Part model, mm, in its own coordinate system. Face numbers are marked on the shaded views. A direction names the side the tool comes from. Give positions to 0.01 mm unless a question says otherwise; leave off trailing zeros. Write each loop counter-clockwise with the first axis right and the second up, starting at its lowest first coordinate (ties: lowest second). Pieces come first, ordered by that corner, then holes. Notation, with made-up numbers: M 77,3 L 131,3 A19 ccw 131,37 Z; hole C -16.5,-38 d10. An arc over 180 degrees is marked long. Write item = value, one per line. Start each with the question number.
from build123d import *

# Parameters (mm, degrees)
EXTRUDE_1_DEPTH     = 20
SKETCH_2_R          = 1.5
EXTRUDE_2_DEPTH     = 4
FILLET_5_R          = 1
CUT_EXTRUDE_1_REACH = 53.828


with BuildPart() as part:
    # 草图1 → 凸台-拉伸1 (new body)
    with BuildSketch(Plane.XY):
        Polygon((20.6, 14), (24.6, 3), (24.6, -2), (20.6, -2), (20.6, 0), (14.6, 0), (14.6, 3), (17.6, 3), (17.6, 6), (14.6, 6), (14.6, 10), (6, 10), (6, 6), (3, 6), (3, 3), (6, 3), (6, 0), (0, 0), (0, 14), align=None)
    extrude(amount=EXTRUDE_1_DEPTH)

    # 草图2 → 凸台-拉伸2 (add)
    with BuildSketch(Plane(origin=(24.6, 0, 0), x_dir=(0, 0, -1), z_dir=(1, 0, 0))):
        with BuildLine():
            Line((-15, -2), (-5, -2))
            Line((-5, -2), (-5, -22))
            ThreePointArc((-5, -22), (-10, -27), (-15, -22))
            Line((-15, -22), (-15, -2))
        make_face()
        with Locations((-10, -22)):
            Circle(SKETCH_2_R, mode=Mode.SUBTRACT)
    extrude(amount=-EXTRUDE_2_DEPTH)

    # 圆角5
    fillet_5_edges = [part.edges().sort_by_distance(p)[0] for p in [
        (16.1, 3, 0),
        (17.6, 4.5, 0),
        (16.1, 6, 0),
        (4.5, 6, 0),
        (3, 4.5, 0),
        (4.5, 3, 0),
        (4.5, 3, 20),
        (3, 4.5, 20),
        (20.6, 14, 10),
        (24.6, 3, 10),
        (4.5, 6, 20),
        (16.1, 6, 20),
        (17.6, 4.5, 20),
        (16.1, 3, 20),
    ]]
    fillet(fillet_5_edges, radius=FILLET_5_R)

    # 草图3 → 切除-拉伸1 (cut, up to next)
    with BuildSketch(Plane(origin=(0, 14, 0), x_dir=(1, 0, 0), z_dir=(0, 1, 0)), mode=Mode.PRIVATE) as cut_extrude_1_sk1:
        with BuildLine():
            Line((8.449786368, -3), (8.449786368, -17))
            ThreePointArc((8.449786368, -17), (9.949786368, -18.5), (11.449786368, -17))
            Line((11.449786368, -17), (11.449786368, -3))
            ThreePointArc((11.449786368, -3), (9.949786368, -1.5), (8.449786368, -3))
        make_face()
    cut_extrude_1_tool1 = extrude(cut_extrude_1_sk1.sketch, amount=-CUT_EXTRUDE_1_REACH, mode=Mode.PRIVATE) & part.part
    add(cut_extrude_1_tool1.solids().sort_by_distance((9.949786, 14, 10))[0], mode=Mode.SUBTRACT)


solid = part.part
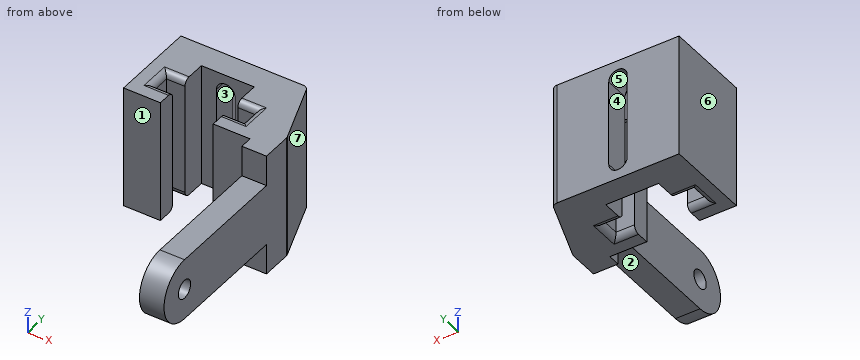
Q1. Tool access for the marked faces 1, 2 and 3: list every direction of +Z, -Z, +X, -X, +Y, -Y with a clear straight run to the whole face (end or side of a thin tool).
Q2. Probe line 1 along Y through (x, z) = (16.25, 17); line 2 along X through (y, z) = (2, 4); line 3 along Y through (x, z) = (7.5, 17). List the from-to ranges inside material, lowest first.
Q3. Drop flat-ended pins along their axis: P1, Ø1.2, axis at x = 22, z = 17.5, coming from the -Y side; P2, Ø1.8, axis at x = 3.5, z = 8.5, coming from the -Y side; P3, Ø2, axis at y = 12.5, z = 12, coming from the -X side; P4, Ø8, axis at x = 7.5, y = -6, coming from the -Z side. Give the stop position or say it passes through.
Q4. Slice it at D-D (z = 13.5). Give the cut face in (x, y), and give its area (3 significant figures).
Q5. Slice it at B-B (z = 10). Give the number of separate pieces and of enclosed holes in the cut face, and give its area (3 significant figures).
Q6. Slice it at C-C (y = 1). Give the cut face in (x, z), and give its area (3 significant figures).
Q7. Slice it at A-A (x = 15.5). Give the cut face in (y, z), and give its area (3 significant figures).
Q8. Two-plate mould, pull along X, no slides. Class the marked faces 4, 5, 6 and 7: +X half, -X half, draft (parallel to the pull), parting line (faces both ways), or undercut.
Working result:
q1.face_1 = +Z, -Z, -X, -Y
q1.face_2 = -Z, +X, -X, -Y
q1.face_3 = +Y, -Y
q2.line_1 = 0 to 3, 6 to 14
q2.line_2 = 0 to 6, 14.6 to 24.6
q2.line_3 = 10 to 14
q3.P1 = -2
q3.P2 = 0
q3.P3 = 0
q3.P4 = through
q4.outline = M 0,0 L 6,0 L 6,3 L 3,3 L 3,6 L 6,6 L 6,10 L 8.45,10 L 8.45,14 L 0,14 Z; M 11.45,10 L 14.6,10 L 14.6,6 L 17.6,6 L 17.6,3 L 14.6,3 L 14.6,0 L 20.6,0 L 20.6,-25.57 L 24.6,-25.57 L 24.6,2.82 A1 ccw 24.54,3.17 L 20.84,13.34 A1 ccw 19.9,14 L 11.45,14 Z
q4.area = 309 mm2
q5.separate_pieces = 3
q5.enclosed_holes = 0
q5.area = 302 mm2
q6.outline = M 0,0 L 6,0 L 6,20 L 0,20 Z; M 14.6,0 L 24.6,0 L 24.6,20 L 14.6,20 Z
q6.area = 320 mm2
q7.outline = M 0,0 L 2,0 A1 ccw 3,1 L 3,19 A1 ccw 2,20 L 0,20 Z; M 6,1 A1 ccw 7,0 L 14,0 L 14,20 L 7,20 A1 ccw 6,19 Z
q7.area = 219 mm2
q8.face_4 = undercut
q8.face_5 = undercut
q8.face_6 = -X half
q8.face_7 = +X half
